Geometry check sheet. Reference: the model listing, model coordinates, mm. A direction names the side the tool comes from. Give positions to 0.01 mm unless a question says otherwise; leave off trailing zeros. Loops run counter-clockwise (first coordinate to the right, second up) from the corner with the lowest first, then second, coordinate; pieces in that order, holes last. Notation, with made-up numbers: (-8, 0.25) -> (18, 0.25) arc R8 cw to (18, 15.25) -> close; hole circle Ø8 at (70.5, 12). An arc over 180 degrees is marked (long way). Write each question's results on one line, items separated by ' | '. Start each with the question number.
1) Draft check along X on faces 4 (the face through (-15, -5, -1)), 5 (the face through (3.078, 0.07, -69.932)), 6 (the face through (-54.43, -0.07, -7.184)), 7 (the face through (7.184, -0.07, 54.43)). Enter one of: pulls with the +X half, pulls with the -X half, needs draft (parallel to the pull), parting line crosses it, or undercut.
2) Depth check by flat-ended pin: pin 1 (8 mm diameter, centred on x = -12.5, z = -54, fed in from -Y); pin 2 (5 mm diameter, centred on x = -12, y = 1, fed in from +Z); pin 3 (2.5 mm diameter, centred on x = -8.23, z = -4.75, fed in from +Y); pin 4 (5 mm diameter, centred on x = -38.5, y = -1.5, fed in from -Z). Enter the tip coordinate at first touch or a pass-through.
3) Set-up check for faces 1 (the face through (-15, 5, -1)), 2 (the face through (54.524, -0.07, 7.302)), 3 (the face through (22.982, 0.023, -55.424)): record each of +Z, -Z, +X, -X, +Y, -Y from which the full face is reachable in a straight line by a thin tool's end or side.
4) Sectioned sample at A-A on z = 0. Record the cut outline in (x, y).
5) Sectioned sample at B-B on x = 0. Record the cut outline in (y, z), then the cut area to 3 significant figures.
6) Sectioned sample at D-D on x = 47. Record the cut outline in (y, z), then the cut area to 3 significant figures.
7) Scan lines: line 1 (X direction, y = -1, z = 9.5); line 2 (X direction, y = -2.75, z = -6.5); line 3 (X direction, y = 2, z = 40). Record each from-to range of solid material in increasing order. Write a range as from..to.
8) Sectioned sample at C-C on z = -45. Record the cut outline in (x, y), then the cut area to 3 significant figures.
```python
from build123d import *

# Parameters (mm, degrees)
SKETCH2_R           = 70
BOSS_EXTRUDE1_DEPTH = 5
CUT_EXTRUDE1_DEPTH  = 10
SKETCH6_R           = 6.1
CUT_EXTRUDE3_DEPTH  = 100.498743711
SKETCH7_R           = 1.7
CUT_EXTRUDE4_DEPTH  = 100.498743711
FILLET1_R           = 6
SKETCH10_R          = 1.65
CUT_EXTRUDE5_DEPTH  = 10
CIRPATTERN2_COUNT   = 8


with BuildPart() as part:
    # Sketch2 → Boss-Extrude1 (new, symmetric)
    with BuildSketch(Plane(origin=(0, 0, 0), x_dir=(1, 0, 0), z_dir=(0, 1, 0))):
        with Locations(Location((0, 0, 0), (0, 0, 270))):
            Circle(SKETCH2_R)
    extrude(amount=BOSS_EXTRUDE1_DEPTH, both=True)

    # Sketch3 → Cut-Extrude1 (cut)
    with BuildSketch(Plane(origin=(0, 5, 0), x_dir=(1, 0, 0), z_dir=(0, 1, 0))):
        with BuildLine():
            Line((-56.780278266, 5), (-16.248076809, 5))
            ThreePointArc((-16.248076809, 5), (-12.02081528, 12.02081528), (-5, 16.248076809))
            Line((-5, 16.248076809), (-5, 56.780278266))
            ThreePointArc((-5, 56.780278266), (-40.305086528, 40.305086528), (-56.780278266, 5))
        make_face()
        with BuildLine():
            ThreePointArc((-56.780278266, -5), (-40.305086528, -40.305086528), (-5, -56.780278266))
            Line((-5, -56.780278266), (-5, -16.248076809))
            ThreePointArc((-5, -16.248076809), (-12.02081528, -12.02081528), (-16.248076809, -5))
            Line((-16.248076809, -5), (-56.780278266, -5))
        make_face()
        with BuildLine():
            Line((5, -16.248076809), (5, -56.780278266))
            ThreePointArc((5, -56.780278266), (40.305086528, -40.305086528), (56.780278266, -5))
            Line((56.780278266, -5), (16.248076809, -5))
            ThreePointArc((16.248076809, -5), (12.02081528, -12.02081528), (5, -16.248076809))
        make_face()
        with BuildLine():
            Line((16.248076809, 5), (56.780278266, 5))
            ThreePointArc((56.780278266, 5), (40.305086528, 40.305086528), (5, 56.780278266))
            Line((5, 56.780278266), (5, 16.248076809))
            ThreePointArc((5, 16.248076809), (12.02081528, 12.02081528), (16.248076809, 5))
        make_face()
    extrude(amount=-CUT_EXTRUDE1_DEPTH, mode=Mode.SUBTRACT)

    # Sketch6 → Cut-Extrude3 (cut, through all)
    with BuildSketch(Plane(origin=(0, 5, 0), x_dir=(1, 0, 0), z_dir=(0, 1, 0))):
        with Locations(Location((0, 0, 0), (0, 0, 270))):
            Circle(SKETCH6_R)
    extrude(amount=-CUT_EXTRUDE3_DEPTH, mode=Mode.SUBTRACT)

    # Sketch7 → Cut-Extrude4 (cut, through all)
    with BuildSketch(Plane(origin=(0, 5, 0), x_dir=(1, 0, 0), z_dir=(0, 1, 0))):
        with Locations(Location((0, 9.5, 0), (0, 0, 270))):
            Circle(SKETCH7_R)
        with Locations(Location((8.227241336, 4.75, 0), (0, 0, 270))):
            Circle(SKETCH7_R)
        with Locations(Location((8.227241336, -4.75, 0), (0, 0, 270))):
            Circle(SKETCH7_R)
        with Locations(Location((0, -9.5, 0), (0, 0, 270))):
            Circle(SKETCH7_R)
        with Locations(Location((-8.227241336, -4.75, 0), (0, 0, 270))):
            Circle(SKETCH7_R)
        with Locations(Location((-8.227241336, 4.75, 0), (0, 0, 270))):
            Circle(SKETCH7_R)
    extrude(amount=-CUT_EXTRUDE4_DEPTH, mode=Mode.SUBTRACT)

    # Fillet1
    fillet1_edges = [part.edges().sort_by_distance(p)[0] for p in [
        (16.248076809, 0, -5),
        (5, 0, -16.248076809),
        (5, 0, -56.780278266),
        (56.780278266, 0, -5),
        (5, 0, 16.248076809),
        (16.248076809, 0, 5),
        (56.780278266, 0, 5),
        (5, 0, 56.780278266),
        (-16.248076809, 0, 5),
        (-5, 0, 16.248076809),
        (-5, 0, 56.780278266),
        (-56.780278266, 0, 5),
        (-5, 0, -16.248076809),
        (-16.248076809, 0, -5),
        (-56.780278266, 0, -5),
        (-5, 0, -56.780278266),
    ]]
    fillet(fillet1_edges, radius=FILLET1_R)

    # Sketch10 → Cut-Extrude5 (cut)
    with BuildSketch(Plane(origin=(64.671567276, 0, -26.787840266), x_dir=(-0.38268343236509067, 0, -0.9238795325112864), z_dir=(0.9238795325112864, 0, -0.38268343236509067))):
        Circle(SKETCH10_R)
    cut_extrude5 = extrude(amount=-CUT_EXTRUDE5_DEPTH, mode=Mode.SUBTRACT)

    # CirPattern2: Cut-Extrude5 ×8 about axis
    cirpattern2_axis = Axis((0, 0, 0), (0, 1, 0))
    for i in range(1, CIRPATTERN2_COUNT):
        add(cut_extrude5.rotate(cirpattern2_axis, i * 360 / CIRPATTERN2_COUNT), mode=Mode.SUBTRACT)


solid = part.part
```
Result:
1) face 4: needs draft | face 5: parting line crosses it | face 6: undercut | face 7: undercut
2) pin 1: y = -5 | pin 2: z = 69.35 | pin 3: through | pin 4: z = -60.03
3) face 1: +Z, -Z, +X, -X, +Y | face 2: +Y, -Y | face 3: none
4) outline: (-70, -5) -> (-6.1, -5) -> (-6.1, 5) -> (-70, 5) -> close; (6.1, -5) -> (70, -5) -> (70, 5) -> (6.1, 5) -> close
5) outline: (-5, -70) -> (5, -70) -> (5, -11.2) -> (-5, -11.2) -> close; (-5, -7.8) -> (5, -7.8) -> (5, -6.1) -> (-5, -6.1) -> close; (-5, 6.1) -> (5, 6.1) -> (5, 7.8) -> (-5, 7.8) -> close; (-5, 11.2) -> (5, 11.2) -> (5, 70) -> (-5, 70) -> close | area: 1,210 mm^2
6) outline: (-5, -51.87) -> (5, -51.87) -> (5, -32.25) -> (-5, -32.25) -> close; (-5, -5) -> (5, -5) -> (5, 5) -> (-5, 5) -> close; (-5, 32.25) -> (5, 32.25) -> (5, 51.87) -> (-5, 51.87) -> close | area: 493 mm^2
7) line 1: -69.35..-55.61, -14.1..-1.7, 1.7..14.1, 55.61..69.35 | line 2: -69.7..-53.77, -16.23..16.23, 53.77..69.7 | line 3: -57.45..-40.61, -5..5, 40.61..57.45
8) outline: (-53.62, -5) -> (-34.99, -5) -> (-34.99, 5) -> (-53.62, 5) -> close; (-5, -5) -> (5, -5) -> (5, 5) -> (-5, 5) -> close; (34.99, -5) -> (53.62, -5) -> (53.62, 5) -> (34.99, 5) -> close | area: 473 mm^2
